from build123d import *

# Parameters (mm, degrees)
SKETCH1_R           = 1.95
SKETCH1_R_2         = 1.45
BOSS_EXTRUDE1_DEPTH = 3


with BuildPart() as part:
    # Sketch1 → Boss-Extrude1 (new body)
    with BuildSketch(Plane.XZ):
        with BuildLine():
            Line((32, 2.95), (-9, 2.95))
            ThreePointArc((-9, 2.95), (-11.95, 0), (-9, -2.95))
            Line((-9, -2.95), (32, -2.95))
            ThreePointArc((32, -2.95), (34.95, 0), (32, 2.95))
        make_face()
        with Locations((32, 0)):
            Circle(SKETCH1_R, mode=Mode.SUBTRACT)
        with Locations((-9, 0)):
            Circle(SKETCH1_R_2, mode=Mode.SUBTRACT)
    extrude(amount=-BOSS_EXTRUDE1_DEPTH)


solid = part.part
Design review of the part built by this model. Coordinates are the model's own, in mm. Give positions to 0.01 mm unless a question says otherwise; leave off trailing zeros. Write each loop counter-clockwise with the first axis right and the second up, starting at its lowest first coordinate (ties: lowest second). Pieces come first, ordered by that corner, then holes. Notation, with made-up numbers: M 38,81 L 56,81 A28 cw 56,117 Z; hole C -2,-35.75 d3. An arc over 180 degrees is marked long. Return JSON: item names as keys, results as strings. Group by question number.
Item 1: The part is to be moulded in two halves that separate along X. For faces 1 (the flat face through (11, 3, 0)), 2 (the cylindrical face through (34.95, 1.48, -0.06)), 3 (the cylindrical face through (33.048, 1.479, 1.644)), say which applies: pulls with the +X half, pulls with the -X half, needs draft (parallel to the pull), parting line crosses it, or undercut.
Item 2: Take a section at C-C (z = 0). Give the boundary of the cut face in (x, y), plus the area to 3 significant figures.
Item 3: Take a section at B-B (y = 0.85). Give the boundary of the cut face in (x, z).
Item 4: Wall thickness on line 1 along X through (y, z) = (1.6, 0.6); line 2 along Z through (x, y) = (32, 0.9); line 3 along X through (y, z) = (2.8, -0.8): over which ranges is each line inside the solid? List them lowest first.
Item 5: Take a section at A-A (x = -8). Give the boundary of the cut face in (y, z), plus the area to 3 significant figures.
Item 6: Clearance check with a flat-ended pin moving along its axis: pin 1 Ø2.5 at (x, z) = (32, 0) entering from +Y. State where the tip first meets the part, or that it passes through.
Return value:
{
 "1": {"face 1": "needs draft", "face 2": "pulls with the +X half", "face 3": "undercut"},
 "2": {"outline": "M -11.95,0 L -10.45,0 L -10.45,3 L -11.95,3 Z; M -7.55,0 L 30.05,0 L 30.05,3 L -7.55,3 Z; M 33.95,0 L 34.95,0 L 34.95,3 L 33.95,3 Z", "area": "120 mm2"},
 "3": {"outline": "M -9,-2.95 L 32,-2.95 A2.95 ccw 32,2.95 L -9,2.95 A2.95 ccw Z; hole C -9,0 d2.9; hole C 32,0 d3.9"},
 "4": {"line 1": "x = -11.89 to -10.32, -7.68 to 30.14, 33.86 to 34.89", "line 2": "z = -2.95 to -1.95, 1.95 to 2.95", "line 3": "x = -11.84 to -10.21, -7.79 to 30.22, 33.78 to 34.84"},
 "5": {"outline": "M 0,-2.95 L 3,-2.95 L 3,-1.05 L 0,-1.05 Z; M 0,1.05 L 3,1.05 L 3,2.95 L 0,2.95 Z", "area": "11.4 mm2"},
 "6": {"pin 1": "passes through"}
}
